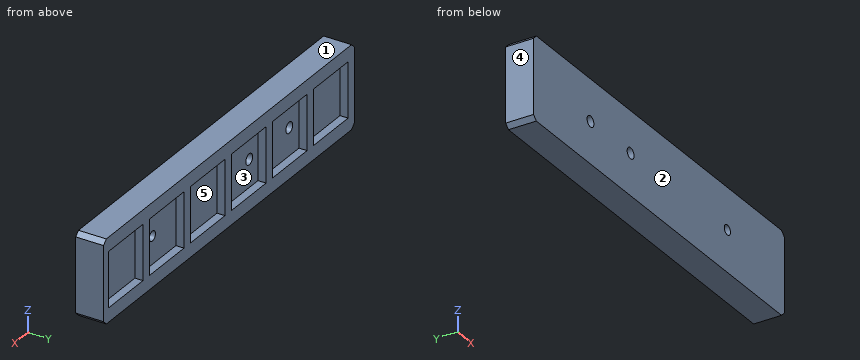
```python
from build123d import *

# Parameters (mm, degrees)
ESBO_O1_W                = 183.2
ESBO_O1_H                = 38.02
RESSALTO_EXTRUS_O1_DEPTH = 12.75
ESBO_O3_W                = 25.34
ESBO_O3_H                = 25.22
CORTE_EXTRUS_O1_DEPTH    = 3.7
CHANFRO1_SIZE            = 2
ESBO_O4_R                = 2.25
ESBO_O4_R_2              = 2.5
CORTE_EXTRUS_O2_DEPTH    = 10100


with BuildPart() as part:
    # Esboço1 → Ressalto-extrusão1 (new body)
    with BuildSketch(Plane(origin=(0, 0, 0), x_dir=(1, 0, 0), z_dir=(0, 1, 0))):
        with Locations((-91.6, 19.01)):
            Rectangle(ESBO_O1_W, ESBO_O1_H)
    extrude(amount=RESSALTO_EXTRUS_O1_DEPTH)

    # Esboço3 → Corte-extrusão1 (cut)
    with BuildSketch(Plane(origin=(0, 12.75, 0), x_dir=(1, 0, 0), z_dir=(0, 1, 0))):
        with Locations((-166.03, 19.01)):
            Rectangle(ESBO_O3_W, ESBO_O3_H)
        with Locations((-136.05, 19.01)):
            Rectangle(ESBO_O3_W, ESBO_O3_H)
        with Locations((-106.07, 19.01)):
            Rectangle(ESBO_O3_W, ESBO_O3_H)
        with Locations((-76.09, 19.01)):
            Rectangle(ESBO_O3_W, ESBO_O3_H)
        with Locations((-46.11, 19.01)):
            Rectangle(ESBO_O3_W, ESBO_O3_H)
        with Locations((-16.13, 19.01)):
            Rectangle(ESBO_O3_W, ESBO_O3_H)
    extrude(amount=-CORTE_EXTRUS_O1_DEPTH, mode=Mode.SUBTRACT)

    # Chanfro1
    chanfro1_edges = [part.edges().sort_by_distance(p)[0] for p in [
        (0, 6.375, 0),
        (-183.2, 6.375, 0),
        (-183.2, 6.375, -38.02),
        (0, 6.375, -38.02),
    ]]
    chamfer(chanfro1_edges, length=CHANFRO1_SIZE)

    # Esboço4 → Corte-extrusão2 (cut)
    with BuildSketch(Plane(origin=(0, 12.75, 0), x_dir=(1, 0, 0), z_dir=(0, 1, 0))):
        with Locations((-41.6, 19.01)):
            Circle(ESBO_O4_R)
        with Locations((-141.6, 19.01)):
            Circle(ESBO_O4_R_2)
        with Locations((-112.310678119, 19.01)):
            Circle(ESBO_O4_R_2)
    extrude(amount=-CORTE_EXTRUS_O2_DEPTH, mode=Mode.SUBTRACT)


solid = part.part
```
Geometry: final body of the model. Coordinates: model frame, mm. Face numbers are marked on the shaded views. A direction names the side the tool comes from. Give positions to 0.01 mm unless a question says otherwise; leave off trailing zeros. Order: outer loops, then holes, each group sorted by start corner. A loop starts at its lowest first (then second) coordinate and runs counter-clockwise, first axis right, second up. Notation, with made-up numbers: M -27,42.5 L -17,42.5 A10 ccw -17,52.5 Z; hole C 39,-36 d1. An arc over 180 degrees is marked long. Answer as CSV lines item,"result". Start each with the question number.
1) Cut plane D-D (z = -19.01). State how many separate pieces and enclosed holes the cut face has, then the cut area to 3 significant figures.
2) Cut plane A-A (x = -141.6). Output: boundary loops of the cut face in (y, z).
3) Set-up query: the marked faces 4 and 5. Return all of +Z, -Z, +X, -X, +Y, -Y with unobstructed straight access to the full face (end or side cutting, diameter ignored); none if empty.
4) Mould query, pull axis Z, two halves, no side actions, for the marked faces 1, 2 and 3. Classes: +Z half, -Z half, draft (parallel to the pull), parting line (faces both ways), or undercut.
5) Line query: line 1 (X direction, y = 7, z = -19.01); line 2 (Z direction, x = -41.6, y = 2.75); line 3 (Z direction, x = -141.6, y = 3). Output: solid intervals per line, ascending. Write a range as from..to.
6) Cut plane C-C (x = -104). Output: boundary loops of the cut face in (y, z).
7) Cut plane B-B (z = -11). Output: boundary loops of the cut face in (x, y).
8) First-contact query: P1, Ø7.5, axis at x = -135.5, z = -22.5, coming from the +Y side; P2, Ø3, axis at x = -141.6, z = -19.01, coming from the +Y side. Flat tips, straight axial feed; report the tip coordinate or a pass-through.
Findings below:
1,separate pieces,"4"
1,enclosed holes,"0"
1,area,"1,640 mm²"
2,outline,"M 0,-38.02 L 12.75,-38.02 L 12.75,-31.62 L 9.05,-31.62 L 9.05,-21.51 L 0,-21.51 Z; M 0,-16.51 L 9.05,-16.51 L 9.05,-6.4 L 12.75,-6.4 L 12.75,0 L 0,0 Z"
3,face 4,"+Z, -Z, -X, +Y, -Y"
3,face 5,"+Y"
4,face 1,"+Z half"
4,face 2,"draft"
4,face 3,"undercut"
5,line 1,"x = -183.2..-144.1, -139.1..-114.81, -109.81..-43.85, -39.35..0"
5,line 2,"z = -38.02..-21.26, -16.76..0"
5,line 3,"z = -38.02..-21.51, -16.51..0"
6,outline,"M 0,-38.02 L 12.75,-38.02 L 12.75,-31.62 L 9.05,-31.62 L 9.05,-6.4 L 12.75,-6.4 L 12.75,0 L 0,0 Z"
7,outline,"M -183.2,0 L 0,0 L 0,12.75 L -3.46,12.75 L -3.46,9.05 L -28.8,9.05 L -28.8,12.75 L -33.44,12.75 L -33.44,9.05 L -58.78,9.05 L -58.78,12.75 L -63.42,12.75 L -63.42,9.05 L -88.76,9.05 L -88.76,12.75 L -93.4,12.75 L -93.4,9.05 L -118.74,9.05 L -118.74,12.75 L -123.38,12.75 L -123.38,9.05 L -148.72,9.05 L -148.72,12.75 L -153.36,12.75 L -153.36,9.05 L -178.7,9.05 L -178.7,12.75 L -183.2,12.75 Z"
8,P1,"stops at y = 9.05"
8,P2,"passes through"
